CAD build for the part. Positions are in the model's coordinates, mm. A direction names the side the tool comes from. Give positions to 0.01 mm unless a question says otherwise; leave off trailing zeros. Loops run counter-clockwise (first coordinate to the right, second up) from the corner with the lowest first, then second, coordinate; pieces in that order, holes last. Notation, with made-up numbers: M 5,31.25 L 39,31.25 A18 cw 39,58.25 Z; hole C -15.75,86.5 d4. An arc over 180 degrees is marked long. Answer as CSV lines item,"result".
```python
from build123d import *
from OCP.BRepFilletAPI import BRepFilletAPI_MakeChamfer

# Parameters (mm, degrees)
CROQUIS1_R              = 1.6
SALIENTE_EXTRUIR1_DEPTH = 10
SALIENTE_EXTRUIR2_DEPTH = 30
CROQUIS12_W             = 12.426406872
CROQUIS12_H             = 4.855948251
CORTAR_EXTRUIR7_DEPTH   = 3.5
CROQUIS3_OUTSIDE_W      = 44.076
CROQUIS3_OUTSIDE_H      = 49.076
CROQUIS3_OUTSIDE_R      = 1.6
CORTAR_EXTRUIR1_DEPTH   = 29
CROQUIS4_R              = 10
SALIENTE_EXTRUIR3_DEPTH = 5
CHAFL_N1_SIZE           = 5
CROQUIS6_R              = 1.6
CORTAR_EXTRUIR3_DEPTH   = 10
CROQUIS8_R              = 6
CROQUIS8_R_2            = 1.6
SALIENTE_EXTRUIR4_DEPTH = 1
CHAFL_N2_SIZE           = 1
CROQUIS5_R              = 3
CORTAR_EXTRUIR4_DEPTH   = 33
CHAFL_N3_SIZE           = 1
CHAFL_N3_SIZE2          = 1.000027611
CHAFL_N3_SIZE2_2        = 1.000000257
CHAFL_N3_SIZE2_3        = 0.999999743
CHAFL_N3_SIZE2_4        = 0.999999708
CHAFL_N3_SIZE2_5        = 1.000000292
CHAFL_N3_SIZE2_6        = 0.999968652
CHAFL_N3_SIZE2_7        = 0.999972392
CHAFL_N3_SIZE2_8        = 1.000031351
CORTAR_EXTRUIR5_START   = -5
CORTAR_EXTRUIR5_DEPTH   = 15
CORTAR_EXTRUIR8_DEPTH   = 48.759815826
CHAFL_N4_SIZE           = 1
CORTAR_EXTRUIR6_DEPTH   = 3.5


with BuildPart() as part:
    # Croquis1 → Saliente-Extruir1 (new body)
    with BuildSketch(Plane(origin=(0, 0, 0), x_dir=(1, 0, 0), z_dir=(0, 1, 0))):
        Polygon((-15, -6.213203436), (-15, -20), (15, -20), (15, -6.213203436), (15, 6.213203436), (6.213203436, 15), (-6.213203436, 15), (-15, 6.213203436), align=None)
        with Locations(Location((0, 0, 0), (0, 0, 270))):
            Circle(CROQUIS1_R, mode=Mode.SUBTRACT)
    extrude(amount=SALIENTE_EXTRUIR1_DEPTH)

    # Croquis2 → Saliente-Extruir2 (add)
    with BuildSketch(Plane.ZY.offset(15)):
        Polygon((10, 20), (4.621471258, 30), (-10, 30), (-10, 39), (10, 39), (20, 20.407554966), (20, 10), (10, 10), align=None)
    extrude(amount=-SALIENTE_EXTRUIR2_DEPTH)

    # Croquis12 → Cortar-Extruir7 (cut)
    with BuildSketch(Plane(origin=(0, 0, 10), x_dir=(-1, 0, 0), z_dir=(0, 0, -1))):
        with Locations((0, 12.427974126)):
            Rectangle(CROQUIS12_W, CROQUIS12_H)
    extrude(amount=-CORTAR_EXTRUIR7_DEPTH, mode=Mode.SUBTRACT)

    # Croquis3 outside → Cortar-Extruir1 (cut)
    # profile 1 of 2: a face of its own
    with BuildSketch(Plane(origin=(0, 39, 0), x_dir=(1, 0, 0), z_dir=(0, 1, 0))):
        with Locations((0, -2.5)):
            Rectangle(CROQUIS3_OUTSIDE_W, CROQUIS3_OUTSIDE_H)
        Polygon((-10, -4.142135624), (-9.999502859, -20), (9.999995364, -20), (10, -4.142135624), (10, 4.142135624), (4.142135624, 10), (-4.142135624, 10), (-10, 4.142135624), align=None, mode=Mode.SUBTRACT)
    # profile 2 of 2: a face of its own
    with BuildSketch(Plane(origin=(0, 39, 0), x_dir=(1, 0, 0), z_dir=(0, 1, 0))):
        with Locations(Location((0, 0, 0), (0, 0, 270))):
            Circle(CROQUIS3_OUTSIDE_R)
    extrude(amount=-CORTAR_EXTRUIR1_DEPTH, mode=Mode.SUBTRACT)

    # Croquis4 → Saliente-Extruir3 (add)
    with BuildSketch(Plane(origin=(0, 39, 0), x_dir=(1, 0, 0), z_dir=(0, 1, 0))):
        with Locations(Location((0, 0, 0), (0, 0, 270))):
            Circle(CROQUIS4_R)
    extrude(amount=SALIENTE_EXTRUIR3_DEPTH)

    # Chaflán1
    chafl_n1_edges = [part.edges().sort_by_distance(p)[0] for p in [
        (0, 44, -10),
    ]]
    chamfer(chafl_n1_edges, length=CHAFL_N1_SIZE - 0.0001)  # a hair under: the kernel refuses the full size

    # Croquis6 → Cortar-Extruir3 (cut)
    with BuildSketch(Plane.XZ):
        with Locations(Location((0, 11, 0), (0, 0, 270))):
            Circle(CROQUIS6_R)
        with Locations(Location((7.778174593, 7.778174593, 0), (0, 0, 270))):
            Circle(CROQUIS6_R)
        with Locations(Location((11, 0, 0), (0, 0, 270))):
            Circle(CROQUIS6_R)
        with Locations(Location((7.778174593, -7.778174593, 0), (0, 0, 270))):
            Circle(CROQUIS6_R)
        with Locations(Location((0, -11, 0), (0, 0, 270))):
            Circle(CROQUIS6_R)
        with Locations(Location((-7.778174593, -7.778174593, 0), (0, 0, 270))):
            Circle(CROQUIS6_R)
        with Locations(Location((-11, 0, 0), (0, 0, 270))):
            Circle(CROQUIS6_R)
        with Locations(Location((-7.778174593, 7.778174593, 0), (0, 0, 270))):
            Circle(CROQUIS6_R)
    extrude(amount=-CORTAR_EXTRUIR3_DEPTH, mode=Mode.SUBTRACT)

    # Croquis8 → Saliente-Extruir4 (add)
    with BuildSketch(Plane(origin=(0, 10, 0), x_dir=(1, 0, 0), z_dir=(0, 1, 0))):
        with Locations(Location((0, 0, 0), (0, 0, 270))):
            Circle(CROQUIS8_R)
        with Locations(Location((0, 0, 0), (0, 0, 270))):
            Circle(CROQUIS8_R_2, mode=Mode.SUBTRACT)
    extrude(amount=SALIENTE_EXTRUIR4_DEPTH)

    # Chaflán2
    chafl_n2_edges = [part.edges().sort_by_distance(p)[0] for p in [
        (0, 10, -6),
    ]]
    chamfer(chafl_n2_edges, length=CHAFL_N2_SIZE - 0.0001)  # a hair under: the kernel refuses the full size

    # Croquis5 → Cortar-Extruir4 (cut)
    with BuildSketch(Plane(origin=(0, 44, 0), x_dir=(1, 0, 0), z_dir=(0, 1, 0))):
        with Locations(Location((0, 0, 0), (0, 0, 270))):
            Circle(CROQUIS5_R)
    extrude(amount=-CORTAR_EXTRUIR4_DEPTH, mode=Mode.SUBTRACT)

    # Chaflán3: one chamfer whose edges measure the first distance from different faces: ONE call of the kernel's chamfer builder (chamfer() names one face for all edges)
    chafl_n3_edges_1 = [part.edges().sort_by_distance(p)[0] for p in [
        (10.606601718, 10, -10.606601718),
        (0, 10, -15),
        (-10.606601718, 10, -10.606601718),
        (-15, 10, 6.893398282),
        (15, 10, 6.893398282),
        (15, 5, 20),
        (-15, 5, 20),
        (0, 0, 20),
        (-12.499751429, 10, 20),
        (12.499997682, 10, 20),
    ]]
    chafl_n3_edges_2 = [part.edges().sort_by_distance(p)[0] for p in [
        (-9.999659608, 29.703777483, 15),
    ]]
    chafl_n3_side_2 = [part.faces().sort_by_distance(p)[0] for p in [
        (-9.999745235, 23.826424788, 12.268639946),
    ]]
    chafl_n3_edges_3 = [part.edges().sort_by_distance(p)[0] for p in [
        (9.999996825, 29.703777483, 15),
    ]]
    chafl_n3_side_3 = [part.faces().sort_by_distance(p)[0] for p in [
        (9.999997624, 23.826424788, 12.268639946),
    ]]
    chafl_n3_edges_4 = [part.edges().sort_by_distance(p)[0] for p in [
        (9.999999074, 25, 7.310735629),
    ]]
    chafl_n3_side_4 = [part.faces().sort_by_distance(p)[0] for p in [
        (9.999997624, 23.826424788, 12.268639946),
    ]]
    chafl_n3_edges_5 = [part.edges().sort_by_distance(p)[0] for p in [
        (9.999998287, 15, 10),
    ]]
    chafl_n3_side_5 = [part.faces().sort_by_distance(p)[0] for p in [
        (0.000130269, 16.111309081, 10),
    ]]
    chafl_n3_edges_6 = [part.edges().sort_by_distance(p)[0] for p in [
        (9.999995364, 15.203777483, 20),
    ]]
    chafl_n3_side_6 = [part.faces().sort_by_distance(p)[0] for p in [
        (0.00010087, 9.179654523, 20),
    ]]
    chafl_n3_edges_7 = [part.edges().sort_by_distance(p)[0] for p in [
        (-9.999816357, 15, 10),
    ]]
    chafl_n3_side_7 = [part.faces().sort_by_distance(p)[0] for p in [
        (-9.999745235, 23.826424788, 12.268639946),
    ]]
    chafl_n3_edges_8 = [part.edges().sort_by_distance(p)[0] for p in [
        (-9.999900665, 25, 7.310735629),
    ]]
    chafl_n3_side_8 = [part.faces().sort_by_distance(p)[0] for p in [
        (-9.999745235, 23.826424788, 12.268639946),
    ]]
    chafl_n3_edges_9 = [part.edges().sort_by_distance(p)[0] for p in [
        (-9.999502859, 15.203777483, 20),
    ]]
    chafl_n3_side_9 = [part.faces().sort_by_distance(p)[0] for p in [
        (-9.999745235, 23.826424788, 12.268639946),
    ]]
    chafl_n3 = BRepFilletAPI_MakeChamfer(part.part.solid().wrapped)
    for e in chafl_n3_edges_1:
        chafl_n3.Add(CHAFL_N3_SIZE, e.wrapped)
    for e in chafl_n3_edges_2:
        chafl_n3.Add(CHAFL_N3_SIZE, CHAFL_N3_SIZE2, e.wrapped, chafl_n3_side_2[0].wrapped)  # the first distance lies on this face
    for e in chafl_n3_edges_3:
        chafl_n3.Add(CHAFL_N3_SIZE, CHAFL_N3_SIZE2_2, e.wrapped, chafl_n3_side_3[0].wrapped)  # the first distance lies on this face
    for e in chafl_n3_edges_4:
        chafl_n3.Add(CHAFL_N3_SIZE, CHAFL_N3_SIZE2_3, e.wrapped, chafl_n3_side_4[0].wrapped)  # the first distance lies on this face
    for e in chafl_n3_edges_5:
        chafl_n3.Add(CHAFL_N3_SIZE, CHAFL_N3_SIZE2_4, e.wrapped, chafl_n3_side_5[0].wrapped)  # the first distance lies on this face
    for e in chafl_n3_edges_6:
        chafl_n3.Add(CHAFL_N3_SIZE, CHAFL_N3_SIZE2_5, e.wrapped, chafl_n3_side_6[0].wrapped)  # the first distance lies on this face
    for e in chafl_n3_edges_7:
        chafl_n3.Add(CHAFL_N3_SIZE, CHAFL_N3_SIZE2_6, e.wrapped, chafl_n3_side_7[0].wrapped)  # the first distance lies on this face
    for e in chafl_n3_edges_8:
        chafl_n3.Add(CHAFL_N3_SIZE, CHAFL_N3_SIZE2_7, e.wrapped, chafl_n3_side_8[0].wrapped)  # the first distance lies on this face
    for e in chafl_n3_edges_9:
        chafl_n3.Add(CHAFL_N3_SIZE, CHAFL_N3_SIZE2_8, e.wrapped, chafl_n3_side_9[0].wrapped)  # the first distance lies on this face
    add(Compound.cast(chafl_n3.Shape()), mode=Mode.REPLACE)

    # Croquis9 → Cortar-Extruir5 (cut)
    with BuildSketch(Plane.XZ.offset(CORTAR_EXTRUIR5_START)):
        Polygon((-10.023540191, -5.532808996), (-10.84540104, -8.600035443), (-8.600035443, -10.84540104), (-5.532808995, -10.023540191), (-4.710948146, -6.956313744), (-6.956313744, -4.710948146), align=None)
        Polygon((-3.175426481, -11), (-1.58771324, -13.75), (1.58771324, -13.75), (3.175426481, -11), (1.58771324, -8.25), (-1.58771324, -8.25), align=None)
        Polygon((-11, 3.175426481), (-13.75, 1.58771324), (-13.75, -1.58771324), (-11, -3.175426481), (-8.25, -1.58771324), (-8.25, 1.58771324), align=None)
        Polygon((-5.532808996, 10.023540191), (-8.600035443, 10.84540104), (-10.84540104, 8.600035443), (-10.023540191, 5.532808995), (-6.956313744, 4.710948146), (-4.710948146, 6.956313744), align=None)
        Polygon((3.175426481, 11), (1.58771324, 13.75), (-1.58771324, 13.75), (-3.175426481, 11), (-1.58771324, 8.25), (1.58771324, 8.25), align=None)
        Polygon((10.023540191, 5.532808996), (10.84540104, 8.600035443), (8.600035443, 10.84540104), (5.532808995, 10.023540191), (4.710948146, 6.956313744), (6.956313744, 4.710948146), align=None)
        Polygon((11, -3.175426481), (13.75, -1.58771324), (13.75, 1.58771324), (11, 3.175426481), (8.25, 1.58771324), (8.25, -1.58771324), align=None)
        Polygon((5.532808996, -10.023540191), (8.600035443, -10.84540104), (10.84540104, -8.600035443), (10.023540191, -5.532808995), (6.956313744, -4.710948146), (4.710948146, -6.956313744), align=None)
    extrude(amount=-CORTAR_EXTRUIR5_DEPTH, mode=Mode.SUBTRACT)

    # Croquis13 → Cortar-Extruir8 (cut, through all)
    with BuildSketch(Plane(origin=(0, 10, -10), x_dir=(-1, 0, 0), z_dir=(0, -1, 0))):
        Polygon((-3.175426481, -21), (-1.58771324, -23.75), (1.58771324, -23.75), (3.175426481, -21), (1.58771324, -18.25), (-1.58771324, -18.25), align=None)
    extrude(amount=-CORTAR_EXTRUIR8_DEPTH, mode=Mode.SUBTRACT)

    # Chaflán4
    chafl_n4_edges = [part.edges().sort_by_distance(p)[0] for p in [
        (0, 44, -3),
    ]]
    chamfer(chafl_n4_edges, length=CHAFL_N4_SIZE)

    # Croquis10 → Cortar-Extruir6 (cut)
    with BuildSketch(Plane.XZ):
        Polygon((3.175426481, 0), (1.58771324, 2.75), (-1.58771324, 2.75), (-3.175426481, 0), (-1.58771324, -2.75), (1.58771324, -2.75), align=None)
    extrude(amount=-CORTAR_EXTRUIR6_DEPTH, mode=Mode.SUBTRACT)


solid = part.part
```
Q1. Cut at B-B (z = 16). Write the cut outline in (x, y), and give its area (3 significant figures).
Solution:
outline,"M -15,0 L 15,0 L 15,9 L 14,10 L 10,10 L 10,25.73 L 9,27.84 L -9,27.84 L -10,25.73 L -10,10 L -14,10 L -15,9 Z"
area,"654 mm²"
Q2. Wall check: line 1 (X direction, y = 7.25, z = 0); line 2 (Z direction, x = 7, y = 5.5); line 3 (X direction, y = 2.6, z = 11). Give the ranges that are in metal, low to high. Write a range as [from, to].
Solution:
line 1,"x = [-15, -13.75], [-8.25, -1.6], [1.6, 8.25], [13.75, 15]"
line 2,"z = [-14.21, -10.42], [-4.72, 4.72], [10.42, 20]"
line 3,"x = [-15, -1.6], [1.6, 15]"
Q3. Cut at A-A (x = 12). Write the cut outline in (y, z).
Solution:
outline,"M 0,-9.21 L 9,-9.21 L 10,-7.8 L 10,-2.6 L 5,-2.6 L 5,-1.25 L 0,-1.25 Z; M 0,1.25 L 5,1.25 L 5,2.6 L 10,2.6 L 10,19 L 9,20 L 1,20 L 0,19 Z"
Q4. Mould opens along X. For faces 1 (the flat face through (-9.5, 14.8, 19.5)), 2 (the flat face through (-8.959, 10.728, 10.487)), 3 (the flat face through (0.1, 9.5, -14.5)) say: released by +X, released by -X, zero draft, split by the parting line, or undercut.
Solution:
face 1,"released by -X"
face 2,"undercut"
face 3,"zero draft"
Q5. Cut at C-C (y = 22.5). Write the cut outline in (x, z).
Solution:
outline,"M -10,9.79 L -9,8.66 L -1.82,8.66 L -3.18,11 L -1.59,13.75 L 1.59,13.75 L 3.18,11 L 1.82,8.66 L 9,8.66 L 10,9.79 L 10,17.74 L 9,18.87 L -9,18.87 L -10,17.74 Z"
Q6. Pin check, flat tips, straight feed: P1, Ø1.5, axis at x = 9.5, z = -8.5, coming from the +Y side; P2, Ø6.5, axis at x = 8, z = 8.5, coming from the +Y side; P3, Ø6, axis at x = -11, y = 26, coming from the -Z side. Stop position of each tip, or through.
Solution:
P1,"stops at y = 5"
P2,"stops at y = 40.58"
P3,"stops at z = 5.57"
Q7. Which spindle directions (+Z, -Z, +X, -X, +Y, -Y) get a long thin tool onto all of the face, cutting with end or side? Do faces 4 (the flat face through (9.5, 14.8, 19.5)), 5 (the flat face through (5, 14.856, 12)), 6 (the cylindrical face through (0.07, 2.46, -9.4)), 7 (the flat face through (12.36, 7.46, -2.39)), 8 (the flat face through (-8.468, 7.465, -5.116)). Say none if no direction does.
Solution:
face 4,"+Z, +X, +Y"
face 5,"-Z"
face 6,"-Y"
face 7,"+Y"
face 8,"none"
Q8. Cut at D-D (y = 7). Give the number of separate pieces and of enclosed holes in the cut face, and give its area (3 significant figures).
Solution:
separate pieces,"1"
enclosed holes,"9"
area,"754 mm²"
